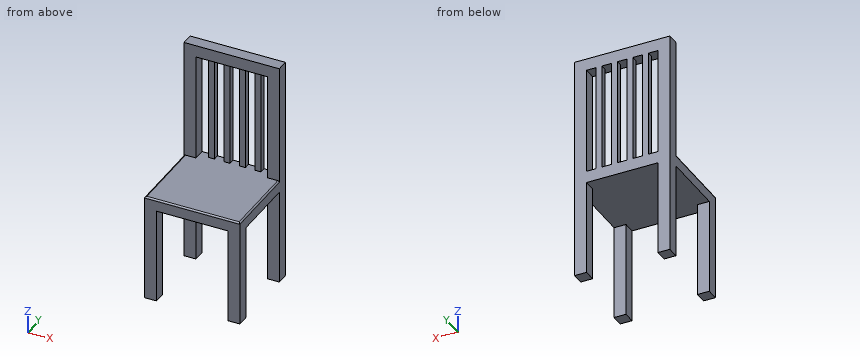
```python
from build123d import *

# Parameters (mm, degrees)
F0_W     = 50.8
F0_H     = 50.8
F1_DEPTH = 406.4
F2_W     = 50.8
F2_H     = 50.8
F3_DEPTH = 50.8
F4_W     = 50.8
F4_H     = 50.8
F4_W_2   = 25.4
F4_H_2   = 25.4
F5_DEPTH = 508
F6_W     = 50.8
F6_H     = 50.8
F7_DEPTH = 355.6
F8_R     = 6.35


with BuildPart() as f1:
    # F0 (on Top) → F1 (new body)
    with BuildSketch(Plane.XY):
        with Locations((-25.4, 25.4)):
            Rectangle(F0_W, F0_H)
        with Locations((330.2, 25.4)):
            Rectangle(F0_W, F0_H)
        with Locations((330.2, -304.8)):
            Rectangle(F0_W, F0_H)
        with Locations((-25.4, -304.8)):
            Rectangle(F0_W, F0_H)
    extrude(amount=F1_DEPTH)

    # F2 (on face) → F3 (join)
    with BuildSketch(Plane.XY.offset(406.4)):
        Polygon((304.8, 0), (304.8, 50.8), (-50.8, 50.8), (-50.8, -330.2), (355.6, -330.2), (355.6, 0), align=None)
        with Locations((330.2, 25.4)):
            Rectangle(F2_W, F2_H)
    extrude(amount=F3_DEPTH)

    # F4 (on face) → F5 (join)
    with BuildSketch(Plane.XY.offset(457.2)):
        with Locations((-25.4, 25.4)):
            Rectangle(F4_W, F4_H)
        with Locations((53.34, 38.1)):
            Rectangle(F4_W_2, F4_H_2)
        with Locations((119.38, 38.1)):
            Rectangle(F4_W_2, F4_H_2)
        with Locations((185.42, 38.1)):
            Rectangle(F4_W_2, F4_H_2)
        with Locations((251.46, 38.1)):
            Rectangle(F4_W_2, F4_H_2)
        with Locations((330.2, 25.4)):
            Rectangle(F4_W, F4_H)
    extrude(amount=F5_DEPTH)

    # F6 (on face) → F7 (join)
    with BuildSketch(Plane.YZ):
        with Locations((25.4, 939.8)):
            Rectangle(F6_W, F6_H)
    extrude(amount=F7_DEPTH)

    # F8
    f8_edges = [f1.edges().sort_by_distance(p)[0] for p in [
        (-50.8, -165.1, 457.2),
        (152.4, -330.2, 457.2),
        (355.6, -165.1, 457.2),
    ]]
    fillet(f8_edges, radius=F8_R)


solid = f1.part
```
Model file for the job. Use its own axes, mm. Round coordinates to 2 decimals unless told otherwise and drop trailing zeros. Loops run counter-clockwise (first coordinate to the right, second up) from the corner with the lowest first, then second, coordinate; pieces in that order, holes last. Notation, with made-up numbers: M 69,41.25 L 77,41.25 A26 cw 77,57.25 Z; hole C 7,-20 d9. An arc over 180 degrees is marked long. Put each result on its own line as item: value. Start each with the question number.
Item 1: Drop flat-ended pins along their axis: P1, Ø7.5, axis at x = 245.5, z = 794.5, coming from the -Y side; P2, Ø4, axis at x = 107, y = -149.5, coming from the +Z side; P3, Ø1, axis at x = 109, y = -128, coming from the -Z side. Give the stop position or say it passes through.
Item 2: Cut at C-C (z = 347). List the corners of the cut face in (x, y), then the cut area to 3 significant figures.
Item 3: Cut at B-B (z = 587). List the corners of the cut face in (x, y), then the cut area to 3 significant figures.
Item 4: Cut at A-A (x = 291.5). List the corners of the cut face in (y, z), then the cut area to 3 significant figures.
Item 5: Cut at D-D (x = 188). List the corners of the cut face in (y, z), then the cut area to 3 significant figures.
Item 6: Drill centre lines: line 1 along X through (y, z) = (33.5, 540); line 2 along X through (y, z) = (11.5, 609.5); line 3 along Y through (x, z) = (192, 605). Where is each one in solid material? Low to high.
Answer block:
1. P1: y = 25.4
1. P2: z = 457.2
1. P3: z = 406.4
2. outline: M -50.8,-330.2 L 0,-330.2 L 0,-279.4 L -50.8,-279.4 Z; M -50.8,0 L 0,0 L 0,50.8 L -50.8,50.8 Z; M 304.8,-330.2 L 355.6,-330.2 L 355.6,-279.4 L 304.8,-279.4 Z; M 304.8,0 L 355.6,0 L 355.6,50.8 L 304.8,50.8 Z
2. area: 10,300 mm2
3. outline: M -50.8,0 L 0,0 L 0,50.8 L -50.8,50.8 Z; M 40.64,25.4 L 66.04,25.4 L 66.04,50.8 L 40.64,50.8 Z; M 106.68,25.4 L 132.08,25.4 L 132.08,50.8 L 106.68,50.8 Z; M 172.72,25.4 L 198.12,25.4 L 198.12,50.8 L 172.72,50.8 Z; M 238.76,25.4 L 264.16,25.4 L 264.16,50.8 L 238.76,50.8 Z; M 304.8,0 L 355.6,0 L 355.6,50.8 L 304.8,50.8 Z
3. area: 7,740 mm2
4. outline: M -330.2,406.4 L 50.8,406.4 L 50.8,457.2 L -323.85,457.2 A6.35 ccw -330.2,450.85 Z; M 0,914.4 L 50.8,914.4 L 50.8,965.2 L 0,965.2 Z
4. area: 21,900 mm2
5. outline: M -330.2,406.4 L 50.8,406.4 L 50.8,965.2 L 0,965.2 L 0,914.4 L 25.4,914.4 L 25.4,457.2 L -323.85,457.2 A6.35 ccw -330.2,450.85 Z
5. area: 33,500 mm2
6. line 1: -50.8 to 0, 40.64 to 66.04, 106.68 to 132.08, 172.72 to 198.12, 238.76 to 264.16, 304.8 to 355.6
6. line 2: -50.8 to 0, 304.8 to 355.6
6. line 3: 25.4 to 50.8
